Verification items for the finished model (mm, model axes). A direction names the side the tool comes from. Round coordinates to 2 decimals unless told otherwise and drop trailing zeros. One line per item, written item: value. Start each with the question number.
Item 1: Draft check along Z on faces 3 (the face through (242, -15, 24)), 4 (the face through (242, 9, -30)), 5 (the face through (242, -12, 0)). Enter one of: +Z half, -Z half, draft (parallel to the pull), parting line (faces both ways), or undercut.
Item 2: Section check A-A, the plane x = 439.5. State how many separate pieces and enclosed holes the cut face has, then the cut area to 3 significant figures.
Item 3: Thickness scan on probe 1 along Z at (x, y) = (407, -9.5); probe 2 along Z at (x, y) = (249.5, 13.5); probe 3 along Z at (x, y) = (350, 10). Record the ranges inside material, lowest first. Write a range as from..to.
Item 4: Tool access check on faces 1 (the face through (242, -15, -24)), 2 (the face through (242, 12, 0)). Record the directions out of +Z, -Z, +X, -X, +Y, -Y that give a thin tool (end or side, any length) a straight path to the whole face; none if there is none.
from build123d import *

# Parameters (mm, degrees)
F0_R     = 3
F1_DEPTH = 490


# Not quite as in the source:
# - ends of sketch curves that miss each other by under 0.0002 mm in the source are joined


with BuildPart() as f1:
    # F0 (on Right) → F1 (new body)
    with BuildSketch(Plane.YZ):
        with BuildLine():
            Line((12.5, -11.85), (15, -11.85))
            Line((15, -11.85), (15, 11.85))
            Line((15, 11.85), (12.5, 11.85))
            Line((12.5, 11.85), (12.5, 9.85))
            Line((12.5, 9.85), (6.547707, 9.85))
            ThreePointArc((6.5477069495, 9.8499999523), (4.5, 15), (6.5477069495, 20.1500000477))
            Line((6.547707, 20.15), (12.5, 20.15))
            Line((12.5, 20.15), (12.5, 18.15))
            Line((12.5, 18.15), (15, 18.15))
            Line((15, 18.15), (15, 30))
            Line((15, 30), (3.15, 30))
            Line((3.15, 30), (3.15, 27.5))
            Line((3.15, 27.5), (5.15, 27.5))
            Line((5.15, 27.5), (5.15, 21.547707))
            ThreePointArc((5.1500000477, 21.5477069495), (0, 19.5), (-5.1500000477, 21.5477069495))
            Line((-5.15, 21.547707), (-5.15, 27.5))
            Line((-5.15, 27.5), (-3.15, 27.5))
            Line((-3.15, 27.5), (-3.15, 30))
            Line((-3.15, 30), (-15, 30))
            Line((-15, 30), (-15, 18.15))
            Line((-15, 18.15), (-12.5, 18.15))
            Line((-12.5, 18.15), (-12.5, 20.15))
            Line((-12.5, 20.15), (-6.547707, 20.15))
            ThreePointArc((-6.5477069495, 20.1500000477), (-4.5, 15), (-6.5477069495, 9.8499999523))
            Line((-6.547707, 9.85), (-12.5, 9.85))
            Line((-12.5, 9.85), (-12.5, 11.85))
            Line((-12.5, 11.85), (-15, 11.85))
            Line((-15, 11.85), (-15, -11.85))
            Line((-15, -11.85), (-12.5, -11.85))
            Line((-12.5, -11.85), (-12.5, -9.85))
            Line((-12.5, -9.85), (-6.547707, -9.85))
            ThreePointArc((-6.5477069495, -9.8499999523), (-4.5, -15), (-6.5477069495, -20.1500000477))
            Line((-6.547707, -20.15), (-12.5, -20.15))
            Line((-12.5, -20.15), (-12.5, -18.15))
            Line((-12.5, -18.15), (-15, -18.15))
            Line((-15, -18.15), (-15, -30))
            Line((-15, -30), (-3.15, -30))
            Line((-3.15, -30), (-3.15, -27.5))
            Line((-3.15, -27.5), (-5.15, -27.5))
            Line((-5.15, -27.5), (-5.15, -21.547707))
            ThreePointArc((-5.1500000477, -21.5477069495), (0, -19.5), (5.1500000477, -21.5477069495))
            Line((5.15, -21.547707), (5.15, -27.5))
            Line((5.15, -27.5), (3.15, -27.5))
            Line((3.15, -27.5), (3.15, -30))
            Line((3.15, -30), (15, -30))
            Line((15, -30), (15, -18.15))
            Line((15, -18.15), (12.5, -18.15))
            Line((12.5, -18.15), (12.5, -20.15))
            Line((12.5, -20.15), (6.547707, -20.15))
            ThreePointArc((6.5477069495, -20.1500000477), (4.5, -15), (6.5477069495, -9.8499999523))
            Line((6.547707, -9.85), (12.5, -9.85))
            Line((12.5, -9.85), (12.5, -11.85))
        make_face()
        with Locations((-10, -25)):
            Circle(F0_R, mode=Mode.SUBTRACT)
        with Locations((10, -25)):
            Circle(F0_R, mode=Mode.SUBTRACT)
        with Locations((-10, 25)):
            Circle(F0_R, mode=Mode.SUBTRACT)
        with BuildLine():
            ThreePointArc((-12, 3.85), (-11.1213203436, 5.9713203436), (-9, 6.85))
            Line((-9, 6.85), (-4.705405, 6.85))
            Line((-4.705405, 6.85), (-1.25, 12.834936))
            ThreePointArc((-1.25, 12.834936), (0, 17.5), (1.2499997876, 12.8349363679))
            Line((1.2499997876, 12.8349363679), (4.705405, 6.85))
            Line((4.705405, 6.85), (9, 6.85))
            ThreePointArc((9, 6.85), (11.1213203436, 5.9713203436), (12, 3.85))
            Line((12, 3.85), (12, -3.85))
            ThreePointArc((12, -3.85), (11.1213203436, -5.9713203436), (9, -6.85))
            Line((9, -6.85), (4.705405, -6.85))
            Line((4.705405, -6.85), (1.25, -12.834937))
            ThreePointArc((1.25, -12.834937), (0, -17.5), (-1.2500002206, -12.8349366179))
            Line((-1.2500002206, -12.8349366179), (-4.705405, -6.85))
            Line((-4.705405, -6.85), (-9, -6.85))
            ThreePointArc((-9, -6.85), (-11.1213203436, -5.9713203436), (-12, -3.85))
            Line((-12, -3.85), (-12, 3.85))
        make_face(mode=Mode.SUBTRACT)
        with Locations((10, 25)):
            Circle(F0_R, mode=Mode.SUBTRACT)
    extrude(amount=F1_DEPTH)


solid = f1.part
Response values:
1. face 3: draft
1. face 4: -Z half
1. face 5: undercut
2. separate pieces: 1
2. enclosed holes: 5
2. area: 707 mm2
3. probe 1: z = -30..-27.96, -22.04..-20.15, -9.85..-6.81, 6.81..9.85, 20.15..22.04, 27.96..30
3. probe 2: z = -30..-18.15, -11.85..11.85, 18.15..30
3. probe 3: z = -30..-28, -22..-20.15, -9.85..-6.68, 6.68..9.85, 20.15..22, 28..30
4. face 1: +Z, -Z, +X, -X, -Y
4. face 2: +X, -X
